Source: CAD feature listing. Evaluate the final solid. Frame: model axes, mm. Face numbers are marked on the shaded views. A direction names the side the tool comes from. Coordinates: 2 decimals unless noted, no trailing zeros. Write each loop counter-clockwise with the first axis right and the second up, starting at its lowest first coordinate (ties: lowest second). Pieces come first, ordered by that corner, then holes. Notation, with made-up numbers: M 24.5,57.25 L 68.5,57.25 A21 cw 68.5,65.25 Z; hole C 3.25,57.5 d3. An arc over 180 degrees is marked long. Write item = value, one per line. Start each with the question number.
1. Section query B-B (y = 6.75). Output: boundary loops of the cut face in (x, z).
2. Section query A-A (x = 0). Output: boundary loops of the cut face in (y, z).
3. Line query: line 1 along X through (y, z) = (8.2, 14); line 2 along Z through (x, y) = (-9.5, 8.3); line 3 along X through (y, z) = (10.25, 13). Output: solid intervals per line, ascending.
4. Section query C-C (z = 2). Output: boundary loops of the cut face in (x, y), then the cut area to 3 significant figures.
5. Pull-direction query (Z, two-part tool) for the marked faces 5, 6, 7 and 8; classes: pulls with the +Z half, pulls with the -Z half, needs draft (parallel to the pull), parting line crosses it, or undercut.
6. Pin query (flat end, axial travel): pin 1 Ø4 at (x, y) = (-10, 5) entering from -Z; pin 2 Ø1.5 at (y, z) = (2.5, -2.5) entering from -X; pin 3 Ø4 at (y, z) = (1.5, -9.5) entering from +X; pin 4 Ø2 at (x, z) = (9, -2.5) entering from -Y. Return the tip coordinate at first contact, or that it passes through.
7. Section query D-D (y = 4.25). Output: boundary loops of the cut face in (x, z).
8. Access query for the marked faces 1, 2, 3 and 4. Directions: +Z, -Z, +X, -X, +Y, -Y. A direction counts if a zero-diameter tool reaches every point of the face in a straight line with its end or side. Return the directions, or none.
```python
from build123d import *

# Parameters (mm, degrees)
SKETCH_1_W          = 15
SKETCH_1_H          = 40
EXTRUDE_1_DEPTH     = 5
SKETCH_2_W          = 26
SKETCH_2_H          = 12
SKETCH_2_R          = 2.5
EXTRUDE_2_DEPTH     = 6
SKETCH_3_W          = 13
SKETCH_3_H          = 9
CUT_EXTRUDE_1_DEPTH = 5


with BuildPart() as part:
    # 草圖1 → 填料-伸長1 (new body)
    with BuildSketch(Plane(origin=(0, 0, 0), x_dir=(1, 0, 0), z_dir=(0, 1, 0))):
        Rectangle(SKETCH_1_W, SKETCH_1_H)
        with BuildLine():
            Line((2.5, 16.799309419), (2.5, -11.700690581))
            ThreePointArc((2.5, -11.700690581), (0, -14.200690581), (-2.5, -11.700690581))
            Line((-2.5, -11.700690581), (-2.5, 16.799309419))
            ThreePointArc((-2.5, 16.799309419), (0, 19.299309419), (2.5, 16.799309419))
        make_face(mode=Mode.SUBTRACT)
    extrude(amount=EXTRUDE_1_DEPTH)

    # 草圖2 → 填料-伸長2 (add)
    with BuildSketch(Plane(origin=(0, 5, 0), x_dir=(1, 0, 0), z_dir=(0, 1, 0))):
        with Locations((0, -14)):
            Rectangle(SKETCH_2_W, SKETCH_2_H)
        with Locations(Location((-9.5, -14, 0), (0, 0, 36.869897646))):
            Circle(SKETCH_2_R, mode=Mode.SUBTRACT)
        with Locations(Location((9.5, -14, 0), (0, 0, 90))):
            Circle(SKETCH_2_R, mode=Mode.SUBTRACT)
    extrude(amount=EXTRUDE_2_DEPTH)

    # 草圖3 → 除料-伸長1 (cut)
    with BuildSketch(Plane(origin=(0, 11, 0), x_dir=(1, 0, 0), z_dir=(0, 1, 0))):
        with Locations((0.015491802, -15.5)):
            Rectangle(SKETCH_3_W, SKETCH_3_H)
    extrude(amount=-CUT_EXTRUDE_1_DEPTH, mode=Mode.SUBTRACT)


solid = part.part
```
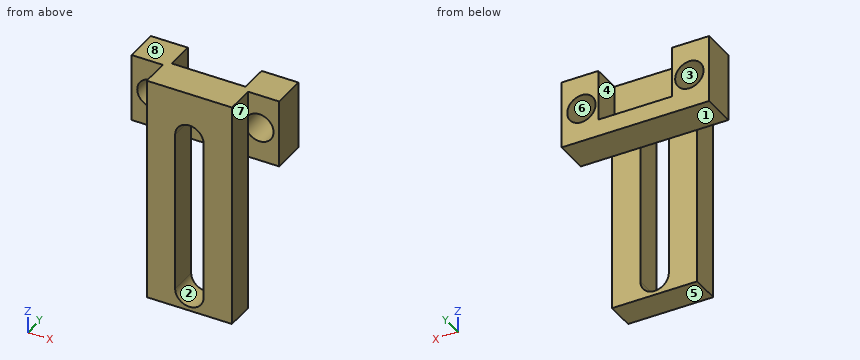
Results are:
q1.outline = M -13,8 L 13,8 L 13,20 L 6.52,20 L 6.52,11 L -6.48,11 L -6.48,20 L -13,20 Z; hole C -9.5,14 d5; hole C 9.5,14 d5
q2.outline = M 0,-20 L 5,-20 L 5,-19.3 L 0,-19.3 Z; M 0,14.2 L 5,14.2 L 5,8 L 11,8 L 11,11 L 6,11 L 6,20 L 0,20 Z
q3.line_1 = -13 to -12, -7 to -6.48, 6.52 to 7, 12 to 13
q3.line_2 = 8 to 11.5, 16.5 to 20
q3.line_3 = -13 to -11.79, -7.21 to -6.48, 6.52 to 7.21, 11.79 to 13
q4.outline = M -7.5,0 L -2.5,0 L -2.5,5 L -7.5,5 Z; M 2.5,0 L 7.5,0 L 7.5,5 L 2.5,5 Z
q4.area = 50.0 mm^2
q5.face_5 = pulls with the -Z half
q5.face_6 = undercut
q5.face_7 = needs draft
q5.face_8 = pulls with the +Z half
q6.pin_1 = 8
q6.pin_2 = -7.5
q6.pin_3 = 7.5
q6.pin_4 = through
q7.outline = M -7.5,-20 L 7.5,-20 L 7.5,20 L -7.5,20 Z; hole M -2.5,-16.8 A2.5 ccw 2.5,-16.8 L 2.5,11.7 A2.5 ccw -2.5,11.7 Z
q8.face_1 = -Z, +X, -X, +Y
q8.face_2 = +Y, -Y
q8.face_3 = +Y
q8.face_4 = +Z, +Y
